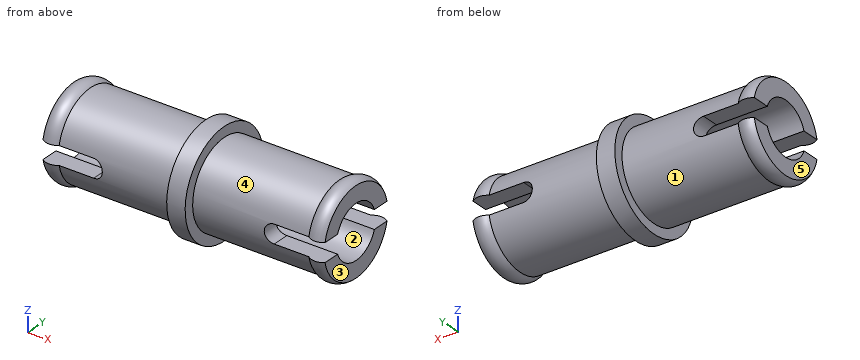
```python
from build123d import *

# Parameters (mm, degrees)
SKETCH1_R           = 2.3622
BASE_EXTRUDE_DEPTH  = 7.239
SKETCH3_R           = 2.921
BOSS_EXTRUDE1_DEPTH = 1.016
SKETCH4_R           = 2.3876
BOSS_EXTRUDE2_DEPTH = 7.239
SKETCH7_R           = 1.4605
CUT_EXTRUDE2_DEPTH  = 17.035227504
CUT_EXTRUDE4_DEPTH  = 10.230899667


with BuildPart() as part:
    # Sketch1 → Base-Extrude (new body)
    with BuildSketch(Plane(origin=(0, 0, 0), x_dir=(0, 0, -1), z_dir=(1, 0, 0))):
        Circle(SKETCH1_R)
    extrude(amount=BASE_EXTRUDE_DEPTH)

    # Sketch3 → Boss-Extrude1 (add)
    with BuildSketch(Plane.ZY):
        Circle(SKETCH3_R)
    extrude(amount=BOSS_EXTRUDE1_DEPTH)

    # Sketch4 → Boss-Extrude2 (add)
    with BuildSketch(Plane.ZY.offset(1.016)):
        Circle(SKETCH4_R)
    extrude(amount=BOSS_EXTRUDE2_DEPTH)

    # Sketch6 → Boss-Revolve2 (revolve)
    with BuildSketch(Plane(origin=(0, 0, 0), x_dir=(1, 0, 0), z_dir=(0, 1, 0)), mode=Mode.PRIVATE) as boss_revolve2_sk:
        with BuildLine():
            Line((-8.255, 2.3876), (-7.366, 2.3876))
            ThreePointArc((-7.366, 2.3876), (-7.8105, 2.54), (-8.255, 2.3876))
        make_face()
    revolve(boss_revolve2_sk.sketch.rotate(Axis((0, 0, 0), (-1, 0, 0)), 180), axis=Axis((0, 0, 0), (-1, 0, 0)))

    # Sketch9 → Boss-Revolve3 (revolve)
    with BuildSketch(Plane(origin=(0, 0, 0), x_dir=(1, 0, 0), z_dir=(0, 1, 0)), mode=Mode.PRIVATE) as boss_revolve3_sk:
        with BuildLine():
            Line((6.35, 2.3622), (7.239, 2.3622))
            ThreePointArc((7.239, 2.3622), (6.7945, 2.520115861), (6.35, 2.3622))
        make_face()
    revolve(boss_revolve3_sk.sketch.rotate(Axis((0, 0, 0), (1, 0, 0)), 180), axis=Axis((0, 0, 0), (1, 0, 0)))

    # Sketch7 → Cut-Extrude2 (cut, through all)
    with BuildSketch(Plane.ZY.offset(8.255)):
        Circle(SKETCH7_R)
    extrude(amount=-CUT_EXTRUDE2_DEPTH, mode=Mode.SUBTRACT)

    # Sketch8 → Cut-Extrude4 (cut, symmetric)
    with BuildSketch(Plane(origin=(0, 0, 0), x_dir=(1, 0, 0), z_dir=(0, 1, 0))):
        with BuildLine():
            Line((-8.255, 0.508), (-5.461, 0.508))
            ThreePointArc((-5.461, 0.508), (-4.953, 0), (-5.461, -0.508))
            Line((-5.461, -0.508), (-8.255, -0.508))
            Line((-8.255, -0.508), (-8.255, 0.508))
        make_face()
    cut_extrude4 = extrude(amount=CUT_EXTRUDE4_DEPTH, both=True, mode=Mode.SUBTRACT)

    # Mirror7: Cut-Extrude4 across plane
    add(cut_extrude4.mirror(Plane(origin=(-0.508, 0, 0), x_dir=(0, 0, 1), z_dir=(1, 0, 0))), mode=Mode.SUBTRACT)


solid = part.part
```
The model under review builds one solid part; all positions refer to its coordinate system, in mm. Face numbers are marked on the shaded views. A direction names the side the tool comes from. Coordinates: 2 decimals unless noted, no trailing zeros. Order: outer loops, then holes, each group sorted by start corner. A loop starts at its lowest first (then second) coordinate and runs counter-clockwise, first axis right, second up. Notation, with made-up numbers: (-40, -3) -> (-28, -3) arc R27 ccw to (-28, 35) -> close; hole circle Ø9 at (64.5, 5). An arc over 180 degrees is marked (long way). Answer in a Markdown table with one row per item. Add a question column.
Item 1: Machinability: for the marked faces 4 and 5, which of the approach directions +Z, -Z, +X, -X, +Y, -Y give a long, thin tool a straight path to every point of the face, cutting with its end or side? Answer none if there is none.
Item 2: Mouldability with a two-part tool opening along Z and no side actions: class the marked faces 1, 2 and 3 as +Z half, -Z half, draft (parallel to the pull), parting line (faces both ways), or undercut.
Item 3: To check wall thickness, follow probe 1 along Y at (x, z) = (-2.5, 0); probe 2 along Y at (x, z) = (6.75, 0.85). State the ranges of each line that lie inside material, in increasing order.
Item 4: We need section C-C on x = -3.75. Write out the cut boundary in (y, z), plus the area to 3 significant figures.
Item 5: We need section A-A on z = 0. Write out the cut boundary in (x, y).
Item 6: Clearance check with flat-ended pins moving along their axes: pin 1 (3 mm diameter, centred on x = 4, y = -2, fed in from -Z); pin 2 (1.5 mm diameter, centred on x = -6, y = -0.5, fed in from -Z); pin 3 (0.6 mm diameter, centred on x = -6.5, y = 2, fed in from +Z). State where each tip first meets the part, or that it passes through.
Final values:
| question | item | result |
|---|---|---|
| 1 | face 4 | none |
| 1 | face 5 | +Z, -Z, -X, +Y, -Y |
| 2 | face 1 | parting line |
| 2 | face 2 | undercut |
| 2 | face 3 | draft |
| 3 | probe 1 | y = -2.39 to -1.46, 1.46 to 2.39 |
| 3 | probe 2 | y = -2.37 to -1.19, 1.19 to 2.37 |
| 4 | outline | circle Ø4.78 at (0, 0); hole circle Ø2.92 at (0, 0) |
| 4 | area | 11.2 mm2 |
| 5 | outline | (-4.95, -2.39) -> (-1.02, -2.39) -> (-1.02, -2.92) -> (0, -2.92) -> (0, -2.36) -> (3.94, -2.36) -> (3.94, -1.46) -> (-4.95, -1.46) -> close; (-4.95, 1.46) -> (3.94, 1.46) -> (3.94, 2.36) -> (0, 2.36) -> (0, 2.92) -> (-1.02, 2.92) -> (-1.02, 2.39) -> (-4.95, 2.39) -> close |
| 6 | pin 1 | stops at z = -2.31 |
| 6 | pin 2 | stops at z = -2.39 |
| 6 | pin 3 | stops at z = 1.68 |
